CAD build for the part. Positions are in the model's coordinates, mm. A direction names the side the tool comes from. Give positions to 0.01 mm unless a question says otherwise; leave off trailing zeros. Loops run counter-clockwise (first coordinate to the right, second up) from the corner with the lowest first, then second, coordinate; pieces in that order, holes last. Notation, with made-up numbers: (73.5, 28.25) - (107.5, 28.25) arc R38 ccw to (107.5, 66.25) - close; hole circle Ø7 at (81.25, 55). An arc over 180 degrees is marked (long way). Return JSON: item names as keys, results as strings.
from build123d import *

# Parameters (mm, degrees)
F0_W     = 20
F0_H     = 20
F1_DEPTH = 20
F2_W     = 12
F2_H     = 12
F3_DEPTH = 25
F4_W     = 12
F4_H     = 12
F5_DEPTH = 25
F6_W     = 12
F6_H     = 12
F7_DEPTH = 25
F8_R     = 0.5
F9_R     = 0.5
F10_R    = 0.5
F11_R    = 0.5
F12_R    = 0.5


with BuildPart() as f1:
    # F0 (on Top) → F1 (new body)
    with BuildSketch(Plane.XY):
        with Locations((1.090192, 0.044756)):
            Rectangle(F0_W, F0_H)
    extrude(amount=F1_DEPTH)

    # F2 (on face) → F3 (cut)
    with BuildSketch(Plane.XY.offset(20)):
        with Locations((1.090192, 0.044756)):
            Rectangle(F2_W, F2_H)
    extrude(amount=-F3_DEPTH, mode=Mode.SUBTRACT)

    # F4 (on face) → F5 (cut)
    with BuildSketch(Plane.YZ.offset(11.090192)):
        with Locations((0.044756, 10)):
            Rectangle(F4_W, F4_H)
    extrude(amount=-F5_DEPTH, mode=Mode.SUBTRACT)

    # F6 (on face) → F7 (cut)
    with BuildSketch(Plane.XZ.offset(9.955244)):
        with Locations((1.090192, 10)):
            Rectangle(F6_W, F6_H)
    extrude(amount=-F7_DEPTH, mode=Mode.SUBTRACT)

    # F8
    f8_edges = [f1.edges().sort_by_distance(p)[0] for p in [
        (1.090192, -9.955244, 20),
    ]]
    fillet(f8_edges, radius=F8_R)

    # F9
    f9_edges = [f1.edges().sort_by_distance(p)[0] for p in [
        (11.090192, 0.294756, 20),
    ]]
    fillet(f9_edges, radius=F9_R)

    # F10
    f10_edges = [f1.edges().sort_by_distance(p)[0] for p in [
        (-8.909808, -9.955244, 9.75),
    ]]
    fillet(f10_edges, radius=F10_R)

    # F11
    f11_edges = [f1.edges().sort_by_distance(p)[0] for p in [
        (1.090192, -9.955244, 0),
    ]]
    fillet(f11_edges, radius=F11_R)

    # F12
    f12_edges = [f1.edges().sort_by_distance(p)[0] for p in [
        (-8.909808, 10.044756, 10),
    ]]
    fillet(f12_edges, radius=F12_R)


solid = f1.part
1. Drill centre lines: probe 1 along Y at (x, z) = (-6.75, 9.75); probe 2 along X at (y, z) = (0.25, 16.5); probe 3 along Z at (x, y) = (8.25, 4.75). Where is each one in solid material? Low to high.
Values follow:
{"probe 1": "y = -9.96 to -5.96, 6.04 to 10.04", "probe 2": "x = -8.91 to -4.91, 7.09 to 11.09", "probe 3": "z = 0 to 4, 16 to 20"}
2. Drop a flat-ended pin along its axis: P1, Ø1, axis at y = 5, z = 10, coming from the +X side. Give the stop position or say it passes through.
Values follow:
{"P1": "passes through"}
3. Which spindle directions (+Z, -Z, +X, -X, +Y, -Y) get a long thin tool onto all of the face, cutting with end or side? Do faces 4 (the face through (7.09, -8, 10)), 5 (the face through (9, 0, 4)), 6 (the face through (7.09, 0, 18)). Say none if no direction does.
Values follow:
{"face 4": "+Y, -Y", "face 5": "+X, -X", "face 6": "+Z, -Z"}
4. Cut at A-A, the plane y = 2. Write the cut outline in (x, z).
Values follow:
{"outline": "(-8.91, 0.5) arc R0.5 ccw to (-8.41, 0) - (-4.91, 0) - (-4.91, 4) - (-8.91, 4) - close; (-8.91, 16) - (-4.91, 16) - (-4.91, 20) - (-8.41, 20) arc R0.5 ccw to (-8.91, 19.5) - close; (7.09, 0) - (10.59, 0) arc R0.5 ccw to (11.09, 0.5) - (11.09, 4) - (7.09, 4) - close; (7.09, 16) - (11.09, 16) - (11.09, 19.5) arc R0.5 ccw to (10.59, 20) - (7.09, 20) - close"}
5. Pull direction Y, two halves, no side cores. Call faces 1 (the face through (-5.4, 10.045, 9.9)), 2 (the face through (11.09, -0.1, 3.5)), 3 (the face through (9, 0, 16)): +Y half, -Y half, draft (parallel to the pull), parting line (faces both ways), or undercut.
Values follow:
{"face 1": "+Y half", "face 2": "draft", "face 3": "undercut"}
6. Cut at D-D, the plane z = 2.5. Write the cut outline in (x, y).
Values follow:
{"outline": "(-8.91, -9.46) arc R0.5 ccw to (-8.41, -9.96) - (10.59, -9.96) arc R0.5 ccw to (11.09, -9.46) - (11.09, 9.54) arc R0.5 ccw to (10.59, 10.04) - (-8.41, 10.04) arc R0.5 ccw to (-8.91, 9.54) - close; hole (-4.91, -5.96) - (7.09, -5.96) - (7.09, 6.04) - (-4.91, 6.04) - close"}
7. Cut at C-C, the plane x = -7.5. Write the cut outline in (y, z).
Values follow:
{"outline": "(-9.96, 0.5) arc R0.5 ccw to (-9.46, 0) - (9.54, 0) arc R0.5 ccw to (10.04, 0.5) - (10.04, 19.5) arc R0.5 ccw to (9.54, 20) - (-9.46, 20) arc R0.5 ccw to (-9.96, 19.5) - close; hole (-5.96, 4) - (6.04, 4) - (6.04, 16) - (-5.96, 16) - close"}
8. Cut at B-B, the plane z = 10. Write the cut outline in (x, y).
Values follow:
{"outline": "(-8.91, -9.46) arc R0.5 ccw to (-8.41, -9.96) - (-4.91, -9.96) - (-4.91, -5.96) - (-8.91, -5.96) - close; (-8.91, 6.04) - (-4.91, 6.04) - (-4.91, 10.04) - (-8.41, 10.04) arc R0.5 ccw to (-8.91, 9.54) - close; (7.09, -9.96) - (10.59, -9.96) arc R0.5 ccw to (11.09, -9.46) - (11.09, -5.96) - (7.09, -5.96) - close; (7.09, 6.04) - (11.09, 6.04) - (11.09, 9.54) arc R0.5 ccw to (10.59, 10.04) - (7.09, 10.04) - close"}
